Check sheet for the drawn part. Datum: minimum x, y, z corner. Units: mm. A direction names the side the tool comes from. Round coordinates to 2 decimals unless told otherwise and drop trailing zeros. Write each loop counter-clockwise with the first axis right and the second up, starting at its lowest first coordinate (ties: lowest second). Pieces come first, ordered by that corner, then holes.
Item 1: Tool access check on the marked faces 4, 5 and 6. Record the directions out of +Z, -Z, +X, -X, +Y, -Y that give a thin tool (end or side, any length) a straight path to the whole face; none if there is none.
Item 2: Cross-section at A-A on z = 28. Enter the section's corners in (x, y), plus the area to 3 significant figures.
Item 3: Cross-section at D-D on y = 14. Enter the section's corners in (x, z).
Item 4: Cross-section at B-B on y = 3. Enter the section's corners in (x, z).
Item 5: Cross-section at C-C on x = 28. Enter the section's corners in (y, z), plus the area to 3 significant figures.
Item 6: Material ranges on line 1 (Y direction, x = 28, z = 53); line 2 (Z direction, x = 28, y = 20); line 3 (Y direction, x = 45, z = 15.5), recorded low to high.
Item 7: Go/stop test with flat-tipped pins: pin 1 Ø1.5 at (y, z) = (2, 31.5) entering from -X; pin 2 Ø14 at (x, z) = (21, 37.5) entering from +Y; pin 3 Ø12 at (x, y) = (33, 10) entering from -Z; pin 4 Ø1.5 at (y, z) = (11.5, 10) entering from -X. Record where each tip stops, or that it passes through.
Item 8: Release check for a two-part mould opening along Z. For the marked faces 1, 2 and 3 record: +Z half, -Z half, draft (parallel to the pull), parting line (faces both ways), or undercut.
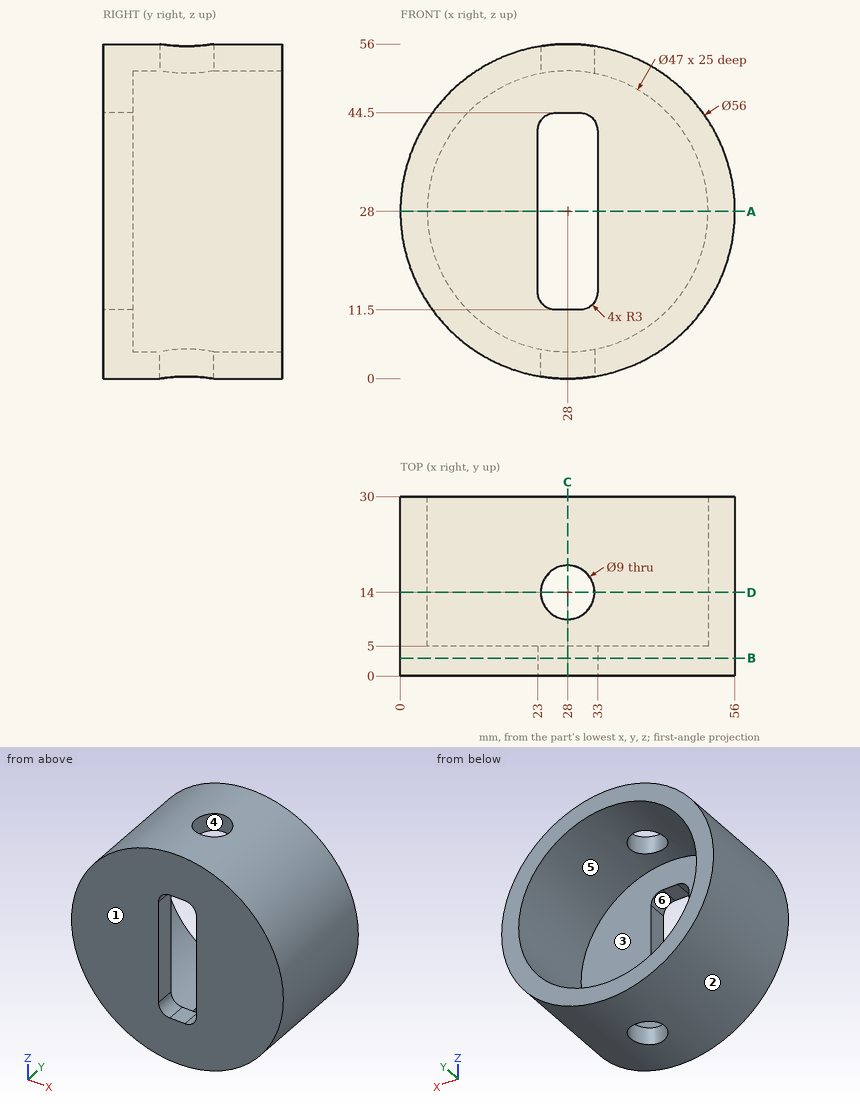
Response values:
1. face 4: +Z, -Z
1. face 5: +Y
1. face 6: +Y, -Y
2. outline: (0, 0) - (23, 0) - (23, 5) - (4.5, 5) - (4.5, 30) - (0, 30) - close; (33, 0) - (56, 0) - (56, 30) - (51.5, 30) - (51.5, 5) - (33, 5) - close
2. area: 455 mm2
3. outline: (23.5, 0.36) - (23.5, 4.93) arc R23.5 cw to (23.5, 51.07) - (23.5, 55.64) arc R28 ccw to start; (32.5, 0.36) arc R28 ccw to (32.5, 55.64) - (32.5, 51.07) arc R23.5 cw to (32.5, 4.93) - close
4. outline: circle Ø56 at (28, 28); hole (23, 14.5) arc R3 ccw to (26, 11.5) - (30, 11.5) arc R3 ccw to (33, 14.5) - (33, 41.5) arc R3 ccw to (30, 44.5) - (26, 44.5) arc R3 ccw to (23, 41.5) - close
5. outline: (0, 0) - (9.5, 0) - (9.5, 4.5) - (5, 4.5) - (5, 11.5) - (0, 11.5) - close; (0, 44.5) - (5, 44.5) - (5, 51.5) - (9.5, 51.5) - (9.5, 56) - (0, 56) - close; (18.5, 0) - (30, 0) - (30, 4.5) - (18.5, 4.5) - close; (18.5, 51.5) - (30, 51.5) - (30, 56) - (18.5, 56) - close
5. area: 259 mm2
6. line 1: y = 0 to 9.5, 18.5 to 30
6. line 2: z = 0 to 4.5, 51.5 to 56
6. line 3: y = 0 to 5
7. pin 1: stops at x = 0.14
7. pin 2: stops at y = 5
7. pin 3: stops at z = 0
7. pin 4: stops at x = 5.94
8. face 1: draft
8. face 2: parting line
8. face 3: undercut
